```python
from build123d import *

# Parameters (mm, degrees)
SKETCH1_W           = 76.2
SKETCH1_H           = 4.7625
BOSS_EXTRUDE1_DEPTH = 152.4
SKETCH2_R           = 4
CUT_EXTRUDE1_DEPTH  = 171.454924852
SKETCH3_W           = 23
SKETCH3_H           = 28
CUT_EXTRUDE2_DEPTH  = 171.454924852
FILLET1_R           = 7.9375
CUT_EXTRUDE3_DEPTH  = 171.454924852
SKETCH5_R           = 1.5
CUT_EXTRUDE4_DEPTH  = 171.454924852
SKETCH6_R           = 3.175
CUT_EXTRUDE5_DEPTH  = 171.454924852
SKETCH7_R           = 3.175
CUT_EXTRUDE6_DEPTH  = 171.454924852


with BuildPart() as part:
    # Sketch1 → Boss-Extrude1 (new body)
    with BuildSketch(Plane(origin=(0, 0, 0), x_dir=(1, 0, 0), z_dir=(0, 1, 0))):
        with Locations((38.1, 2.38125)):
            Rectangle(SKETCH1_W, SKETCH1_H)
    extrude(amount=BOSS_EXTRUDE1_DEPTH)

    # Sketch2 → Cut-Extrude1 (cut, through all)
    with BuildSketch(Plane.XY):
        with Locations((23.5, 42)):
            Circle(SKETCH2_R)
        with Locations((45.5, 78.451705922)):
            Circle(SKETCH2_R)
    extrude(amount=-CUT_EXTRUDE1_DEPTH, mode=Mode.SUBTRACT)

    # Sketch3 → Cut-Extrude2 (cut, through all)
    with BuildSketch(Plane.XY):
        with Locations((23.5, 68)):
            Rectangle(SKETCH3_W, SKETCH3_H)
    extrude(amount=-CUT_EXTRUDE2_DEPTH, mode=Mode.SUBTRACT)

    # Fillet1
    fillet1_edges = [part.edges().sort_by_distance(p)[0] for p in [
        (12, 54, -2.38125),
        (12, 82, -2.38125),
        (35, 82, -2.38125),
        (35, 54, -2.38125),
    ]]
    fillet(fillet1_edges, radius=FILLET1_R)

    # Sketch4 → Cut-Extrude3 (cut, through all)
    with BuildSketch(Plane.XY):
        with BuildLine():
            Line((6.3, 110.451705922), (6.3, 88.451705922))
            ThreePointArc((6.3, 88.451705922), (4.8, 86.951705922), (3.3, 88.451705922))
            Line((3.3, 88.451705922), (3.3, 110.451705922))
            ThreePointArc((3.3, 110.451705922), (4.8, 111.951705922), (6.3, 110.451705922))
        make_face()
        with BuildLine():
            Line((21.3, 110.451705922), (21.3, 88.451705922))
            ThreePointArc((21.3, 88.451705922), (19.8, 86.951705922), (18.3, 88.451705922))
            Line((18.3, 88.451705922), (18.3, 110.451705922))
            ThreePointArc((18.3, 110.451705922), (19.8, 111.951705922), (21.3, 110.451705922))
        make_face()
    extrude(amount=-CUT_EXTRUDE3_DEPTH, mode=Mode.SUBTRACT)

    # Sketch5 → Cut-Extrude4 (cut, through all)
    with BuildSketch(Plane.XY):
        with Locations((5, 36)):
            Circle(SKETCH5_R)
        with Locations((42, 36)):
            Circle(SKETCH5_R)
        with Locations((5, 46)):
            Circle(SKETCH5_R)
        with Locations((42, 46)):
            Circle(SKETCH5_R)
    extrude(amount=-CUT_EXTRUDE4_DEPTH, mode=Mode.SUBTRACT)

    # Sketch6 → Cut-Extrude5 (cut, through all)
    with BuildSketch(Plane.XY):
        with Locations((12.7, 12.7)):
            Circle(SKETCH6_R)
        with Locations((63.5, 12.7)):
            Circle(SKETCH6_R)
    extrude(amount=-CUT_EXTRUDE5_DEPTH, mode=Mode.SUBTRACT)

    # Sketch7 → Cut-Extrude6 (cut, through all)
    with BuildSketch(Plane.XY):
        with Locations((25, 142.4)):
            Circle(SKETCH7_R)
    extrude(amount=-CUT_EXTRUDE6_DEPTH, mode=Mode.SUBTRACT)


solid = part.part
```
Input: part model. Units: mm. Frame: model coordinates. Round coordinates to 2 decimals unless told otherwise and drop trailing zeros. Loops run counter-clockwise (first coordinate to the right, second up) from the corner with the lowest first, then second, coordinate; pieces in that order, holes last. Notation, with made-up numbers: M 76.25,54.5 L 88.25,54.5 A12 cw 88.25,67.5 Z; hole C 5,-33.5 d11. An arc over 180 degrees is marked long. Answer in a Markdown table with one row per item. Add a question column.
1. Section C-C (y = 96). Output: boundary loops of the cut face in (x, z).
2. Section A-A (y = 42). Output: boundary loops of the cut face in (x, z).
3. Section B-B (x = 23.5). Output: boundary loops of the cut face in (y, z).
4. Section D-D (z = -3.75). Give the number of separate pieces and of enclosed holes in the cut face, and give its area (3 significant figures).
5. Ray query, probe 1 along Y at (x, z) = (5, -2.8); probe 2 along X at (y, z) = (107.5, -2.5); probe 3 along Y at (x, z) = (12.7, -1.45) (3 decimals). Return the intervals inside material, ascending.
6. Mould query, pull axis Y, two halves, no side actions, for faces 1 (the face through (38, 152.4, -2)), 2 (the face through (19.77, 111.95, -2.35)), 3 (the face through (0, 75, -2)). Classes: released by +Y, released by -Y, zero draft, split by the parting line, or undercut.
Values follow:
| question | item | result |
|---|---|---|
| 1 | outline | M 0,-4.76 L 3.3,-4.76 L 3.3,0 L 0,0 Z; M 6.3,-4.76 L 18.3,-4.76 L 18.3,0 L 6.3,0 Z; M 21.3,-4.76 L 76.2,-4.76 L 76.2,0 L 21.3,0 Z |
| 2 | outline | M 0,-4.76 L 19.5,-4.76 L 19.5,0 L 0,0 Z; M 27.5,-4.76 L 76.2,-4.76 L 76.2,0 L 27.5,0 Z |
| 3 | outline | M 0,-4.76 L 38,-4.76 L 38,0 L 0,0 Z; M 46,-4.76 L 54,-4.76 L 54,0 L 46,0 Z; M 82,-4.76 L 139.6,-4.76 L 139.6,0 L 82,0 Z; M 145.2,-4.76 L 152.4,-4.76 L 152.4,0 L 145.2,0 Z |
| 4 | separate pieces | 1 |
| 4 | enclosed holes | 12 |
| 4 | area | 10,700 mm^2 |
| 5 | probe 1 | 0 to 34.5, 37.5 to 44.5, 47.5 to 86.97, 111.94 to 152.4 |
| 5 | probe 2 | 0 to 3.3, 6.3 to 18.3, 21.3 to 76.2 |
| 5 | probe 3 | 0 to 9.525, 15.875 to 58.678, 77.322 to 152.4 |
| 6 | face 1 | released by +Y |
| 6 | face 2 | undercut |
| 6 | face 3 | zero draft |
